Source: CAD feature listing. Evaluate the final solid. Frame: model axes, mm. Give positions to 0.01 mm unless a question says otherwise; leave off trailing zeros.
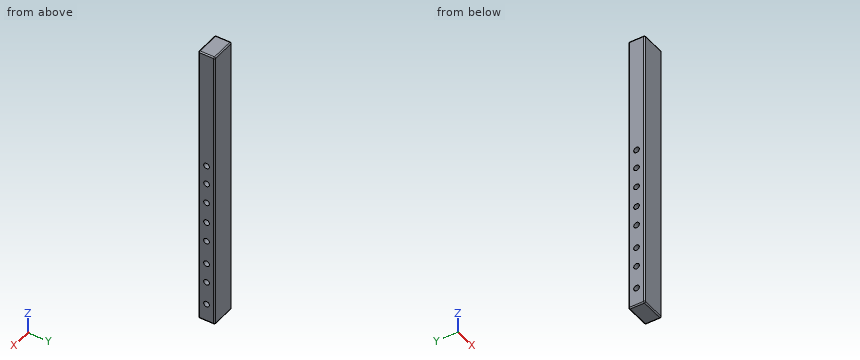
from build123d import *

# Parameters (mm, degrees)
F0_W     = 11.4448349923
F0_H     = 7.429568097
F1_DEPTH = 128.27
F2_R     = 0.508
F4_D     = 2.54
F4_DEPTH = 12.7
F4_TIP   = 0.7630929862
F5_D     = 2.54
F5_DEPTH = 12.7
F5_TIP   = 0.7630929862


with BuildPart() as f1:
    # F0 (on Top) → F1 (new body)
    with BuildSketch(Plane.XY):
        Rectangle(F0_W, F0_H)
    extrude(amount=F1_DEPTH)

    # F2
    f2_edges = [f1.edges().sort_by_distance(p)[0] for p in [
        (-5.722417, 3.714784, 64.135),
        (-5.722417, -3.714784, 64.135),
        (-5.722417, 0, 0),
        (-5.722417, 0, 128.27),
        (5.722417, -3.714784, 64.135),
        (0, -3.714784, 0),
        (0, -3.714784, 128.27),
        (5.722417, 0, 128.27),
        (0, 3.714784, 128.27),
        (5.722417, 3.714784, 64.135),
        (5.722417, 0, 0),
        (0, 3.714784, 0),
    ]]
    fillet(f2_edges, radius=F2_R)

    # F4 (one way)
    with BuildSketch(Plane.YZ):
        with Locations((0, 74.714243412), (0, 66.1139637232), (0, 56.9976679981), (0, 47.5373640656), (0, 38.5930761695), (0, 27.7567245066), (0, 18.8124384731), (0, 8.3200978115)):
            Circle(F4_D / 2)
    extrude(amount=-F4_DEPTH, mode=Mode.SUBTRACT)
    with Locations(Plane.YZ):
        with Locations((0, 74.714243412), (0, 66.1139637232), (0, 56.9976679981), (0, 47.5373640656), (0, 38.5930761695), (0, 27.7567245066), (0, 18.8124384731), (0, 8.3200978115)):
            with Locations((0, 0, -(F4_DEPTH + F4_TIP / 2))):  # 118° drill point
                Cone(0, F4_D / 2, F4_TIP, mode=Mode.SUBTRACT)

    # F5
    with Locations(Plane(origin=(0, 0, 0), x_dir=(0, 1, 0), z_dir=(-1, 0, 0))):
        with Locations((0, -74.714243412), (0, -66.1139637232), (0, -56.9976679981), (0, -47.5373640656), (0, -38.5930761695), (0, -27.7567245066), (0, -18.8124384731), (0, -8.3200978115)):
            Hole(F5_D / 2, depth=F5_DEPTH)
            with Locations((0, 0, -(F5_DEPTH + F5_TIP / 2))):  # 118° drill point
                Cone(0, F5_D / 2, F5_TIP, mode=Mode.SUBTRACT)


solid = f1.part
1) Cut plane A-A (x = -2.5). State how many separate pieces and enclosed holes the cut face has, and give its area (3 significant figures).
Checks:
separate pieces: 1
enclosed holes: 8
area: 912 mm2
2) Ray query, probe 1 along Y at (x, z) = (-1.75, 47.5); probe 2 along X at (y, z) = (3.25, 44); probe 3 along Y at (x, z) = (-1.75, 67). Return the intervals inside material, ascending.
Checks:
probe 1: y = -3.71 to -1.27, 1.27 to 3.71
probe 2: x = -5.72 to 5.72
probe 3: y = -3.71 to -0.91, 0.91 to 3.71
3) Contact query for a flat-ended pin moving along its axis: P1, Ø1, axis at y = -0.5, z = 57, coming from the +X side. Output: stop coordinate, or through.
Checks:
P1: passes through
